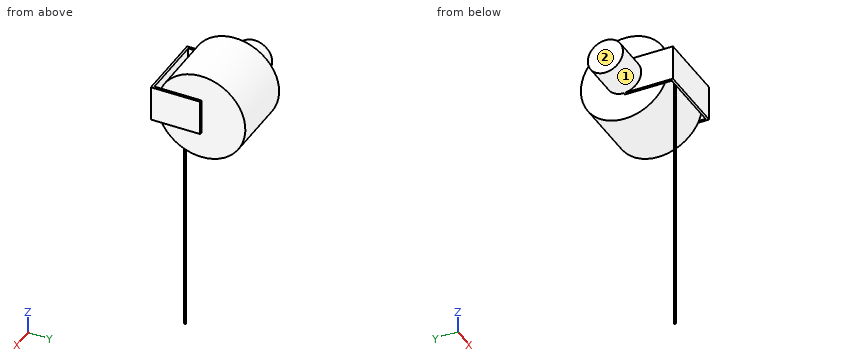
from build123d import *

# Parameters (mm, degrees)
SKETCH1_R           = 187.5
BOSS_EXTRUDE1_DEPTH = 282
SKETCH2_W           = 150
SKETCH2_H           = 210
BOSS_EXTRUDE2_DEPTH = 10
SKETCH3_W           = 150
SKETCH3_H           = 210
BOSS_EXTRUDE3_DEPTH = 10
BOSS_EXTRUDE4_REACH = 294
SKETCH4_W           = 150
SKETCH4_H           = 10
SKETCH5_R           = 75
BOSS_EXTRUDE5_DEPTH = 152.4
SKETCH7_R           = 3.8
SKETCH8_R           = 3.8
BOSS_EXTRUDE6_DEPTH = 967.2


with BuildPart() as part:
    # Sketch1 → Boss-Extrude1 (new body)
    with BuildSketch(Plane(origin=(0, 0, 0), x_dir=(0, 0, -1), z_dir=(1, 0, 0))):
        Circle(SKETCH1_R)
    extrude(amount=BOSS_EXTRUDE1_DEPTH)

    # Sketch2 → Boss-Extrude2 (add)
    with BuildSketch(Plane.ZY):
        with Locations((0, -105)):
            Rectangle(SKETCH2_W, SKETCH2_H)
    extrude(amount=BOSS_EXTRUDE2_DEPTH)

    # Sketch3 → Boss-Extrude3 (add)
    with BuildSketch(Plane(origin=(282, 0, 0), x_dir=(0, 0, -1), z_dir=(1, 0, 0))):
        with Locations((0, -105)):
            Rectangle(SKETCH3_W, SKETCH3_H)
    extrude(amount=BOSS_EXTRUDE3_DEPTH)

    # Sketch4 → Boss-Extrude4 (add, up to next)
    with BuildSketch(Plane(origin=(0, 0, 0), x_dir=(0, 0, -1), z_dir=(1, 0, 0)), mode=Mode.PRIVATE) as boss_extrude4_sk1:
        with Locations((0, -205)):
            Rectangle(SKETCH4_W, SKETCH4_H)
    boss_extrude4_tool1 = extrude(boss_extrude4_sk1.sketch, amount=BOSS_EXTRUDE4_REACH, mode=Mode.PRIVATE) - part.part
    add(boss_extrude4_tool1.solids().sort_by_distance((0, -205, 0))[0])

    # Sketch5 → Boss-Extrude5 (add)
    with BuildSketch(Plane.ZY.offset(10)):
        Circle(SKETCH5_R)
    extrude(amount=BOSS_EXTRUDE5_DEPTH)

    # Sweep1: sweep along a path in Sketch6
    with BuildLine(Plane(origin=(50.7, 0, 0), x_dir=(0, 0, -1), z_dir=(1, 0, 0))) as sweep1_path:
        Line((0, -187.5), (200, -187.5))
    # Sketch7 → Sweep1 (sweep)
    with BuildSketch(Plane(origin=(0, 0, -200), x_dir=(-1, 0, 0), z_dir=(0, 0, -1))):
        with Locations((-50.7, -187.5)):
            Circle(SKETCH7_R)
    sweep(path=sweep1_path.line)

    # Sketch8 → Boss-Extrude6 (add)
    with BuildSketch(Plane(origin=(0, 0, -200), x_dir=(-1, 0, 0), z_dir=(0, 0, -1))):
        with Locations((-50.7, -187.5)):
            Circle(SKETCH8_R)
    extrude(amount=BOSS_EXTRUDE6_DEPTH)


solid = part.part
Part model, mm, in its own coordinate system. Face numbers are marked on the shaded views. A direction names the side the tool comes from. Give positions to 0.01 mm unless a question says otherwise; leave off trailing zeros. Loops run counter-clockwise (first coordinate to the right, second up) from the corner with the lowest first, then second, coordinate; pieces in that order, holes last. Notation, with made-up numbers: M -26,70.5 L 9,70.5 A16 cw 9,95.5 Z; hole C 46,85 d1. An arc over 180 degrees is marked long. Put each result on its own line as item: value. Start each with the question number.
1) Saw through at B-B (y = -51). List the corners of the cut face in (x, z).
2) Saw through at C-C (z = -976.5). List the corners of the cut face in (x, y).
3) 3-axis set-ups, long thin cutter, end or side, ignore diameter. For the marked faces 1 and 2: which of +Z, -Z, +X, -X, +Y, -Y reach the whole face in a straight line?
4) Flat gauge pins, fed straight in: pin 1 (1.5 mm diameter, centred on x = -24.5, y = 37, fed in from +Z); pin 2 (8 mm diameter, centred on x = -65, y = -38, fed in from +Z); pin 3 (3 mm diameter, centred on x = -6.5, z = 28.5, fed in from +Y). Where does each tip first touch, or does it go through?
5) Probe probe 1 along X at (y, z) = (-76, 16); probe 2 along Z at (x, y) = (-79, -46); probe 3 along Z at (x, y) = (-62.5, 63). List the from-to ranges inside material, lowest first.
6) Saw through at D-D (y = -152.5). List the corners of the cut face in (x, z).
7) Saw through at A-A (x = 245). List the corners of the cut face in (y, z).
Numbers:
1. outline: M -162.4,-54.99 L -10,-54.99 L -10,-75 L 0,-75 L 0,-180.43 L 282,-180.43 L 282,-75 L 292,-75 L 292,75 L 282,75 L 282,180.43 L 0,180.43 L 0,75 L -10,75 L -10,54.99 L -162.4,54.99 Z
2. outline: C 50.7,-187.5 d7.6
3. face 1: -X
3. face 2: +Z, -Z, -X, +Y, -Y
4. pin 1: z = 65.66
4. pin 2: z = 66.85
4. pin 3: y = 0
5. probe 1: -10 to 292
5. probe 2: -59.24 to 59.24
5. probe 3: -40.69 to 40.69
6. outline: M -10,-75 L 0,-75 L 0,-109.09 L 282,-109.09 L 282,-75 L 292,-75 L 292,75 L 282,75 L 282,109.09 L 0,109.09 L 0,75 L -10,75 Z
7. outline: M -210,-75 L -200,-75 L -200,75 L -210,75 Z; C 0,0 d375
